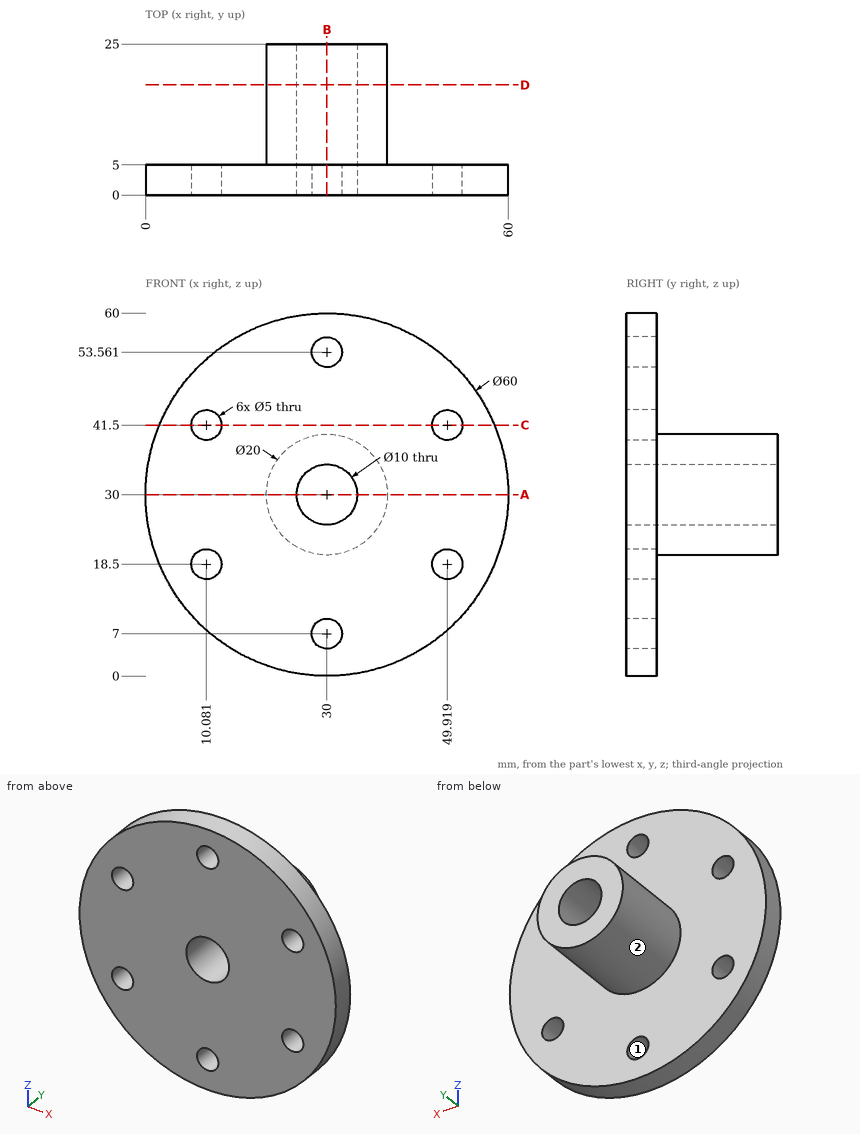
Verification items for this drawing (mm, ordinates from the low corner). A direction names the side the tool comes from. Give positions to 0.01 mm unless a question says otherwise; leave off trailing zeros. Loops run counter-clockwise (first coordinate to the right, second up) from the corner with the lowest first, then second, coordinate; pieces in that order, holes last. Notation, with made-up numbers: M 29,-3.75 L 81,-3.75 A19 cw 81,15.25 Z; hole C 76,-27.75 d2. An arc over 180 degrees is marked long. Return JSON: item names as keys, results as strings. Group by question number.
1. Cross-section at A-A on z = 30. Record the boundary of the cut face in (x, y), plus the area to 3 significant figures.
2. Thickness scan on L1, parallel to Z at x = 30, y = 3.6; L2, parallel to Z at x = 30, y = 8.25; L3, parallel to X at y = 1.5, z = 41. Record the ranges inside material, lowest first.
3. Cross-section at B-B on x = 30. Record the boundary of the cut face in (y, z).
4. Tool access check on the marked faces 1 and 2. Record the directions out of +Z, -Z, +X, -X, +Y, -Y that give a thin tool (end or side, any length) a straight path to the whole face; none if there is none.
5. Cross-section at C-C on z = 41.5. Record the boundary of the cut face in (x, y).
6. Cross-section at D-D on y = 18.25. Record the boundary of the cut face in (x, z), plus the area to 3 significant figures.
7. Go/stop test with flat-tipped pins: pin 1 (8 mm diameter, centred on x = 49.92, z = 41.5, fed in from +Y); pin 2 (10 mm diameter, centred on y = 7.5, z = 13.5, fed in from -X); pin 3 (1 mm diameter, centred on x = 29, y = 17, fed in from +Z). Record where each tip stops, or that it passes through.
Return value:
{
 "1": {"outline": "M 0,0 L 25,0 L 25,25 L 20,25 L 20,5 L 0,5 Z; M 35,0 L 60,0 L 60,5 L 40,5 L 40,25 L 35,25 Z", "area": "450 mm^2"},
 "2": {"L1": "0 to 4.5, 9.5 to 25, 35 to 51.06, 56.06 to 60", "L2": "20 to 25, 35 to 40", "L3": "2.09 to 7.63, 12.53 to 47.47, 52.37 to 57.91"},
 "3": {"outline": "M 0,0 L 5,0 L 5,4.5 L 0,4.5 Z; M 0,9.5 L 5,9.5 L 5,20 L 25,20 L 25,25 L 0,25 Z; M 0,35 L 25,35 L 25,40 L 5,40 L 5,51.06 L 0,51.06 Z; M 0,56.06 L 5,56.06 L 5,60 L 0,60 Z"},
 "4": {"face 1": "+Y, -Y", "face 2": "+Y"},
 "5": {"outline": "M 2.29,0 L 7.58,0 L 7.58,5 L 2.29,5 Z; M 12.58,0 L 47.42,0 L 47.42,5 L 12.58,5 Z; M 52.42,0 L 57.71,0 L 57.71,5 L 52.42,5 Z"},
 "6": {"outline": "C 30,30 d20; hole C 30,30 d10", "area": "236 mm^2"},
 "7": {"pin 1": "y = 5", "pin 2": "x = 2.58", "pin 3": "z = 39.99"}
}
